Source: CAD feature listing. Evaluate the final solid. Frame: model axes, mm. A direction names the side the tool comes from. Round coordinates to 2 decimals unless told otherwise and drop trailing zeros. Order: outer loops, then holes, each group sorted by start corner. A loop starts at its lowest first (then second) coordinate and runs counter-clockwise, first axis right, second up. Notation, with made-up numbers: (10, -33.5) -> (58, -33.5) arc R17 ccw to (58, -4.5) -> close; hole circle Ø5 at (37.5, 16). An arc over 180 degrees is marked (long way). Write item = value, one per line. Start each with the question number.
(1) Cut plane B-B on y = 6. Return the cut outline in (x, z), then the cut area to 3 significant figures.
(2) Reachability of faces 4 (the face through (-16.296, 1.164, 45.286)), 5 (the face through (-7.105, 0.76, 41.004)), 6 (the face through (-4, 14.353, 14)), 7 (the face through (-4, -26.247, 14)), 8 (the face through (-14.208, -6, 19)) from +Z, -Z, +X, -X, +Y, -Y: full face, straight path, thin tool, end or side. Return the list, or none.
(3) Cut plane A-A on x = 1.25. Return the cut outline in (y, z).
(4) Cut plane D-D on z = 29.5. Return the cut outline in (x, y), then the cut area to 3 significant figures.
(5) Ray query, line 1 (Z direction, x = 0.5, y = -9.5); line 2 (Y direction, x = -10, z = 4); line 3 (Z direction, x = -13, y = -16). Return the intervals inside material, ascending.
(6) Cut plane C-C on y = -28.5. Return the cut outline in (x, z).
(7) Draft query along Y for faces 1 (the face through (-2, -2, 44.3)), 2 (the face through (-4, 20.753, 29)), 3 (the face through (1.305, -32.344, 28.972)). Return one class per face: released by +Y, released by -Y, zero draft, split by the parting line, or undercut.
(8) Contact query for flat-ended pins moving along their axis: pin 1 Ø5 at (x, z) = (-7.5, 9.5) entering from -Y; pin 2 Ø6 at (x, y) = (-10.41, 18.25) entering from -Z; pin 3 Ø1.5 at (y, z) = (-14, 34) entering from +X; pin 4 Ø3.5 at (x, y) = (1.79, -30.15) entering from -Z. Output: stop coordinate, or through.
from build123d import *

# Parameters (mm, degrees)
F0_W      = 19.8
F0_H      = 40.6
F1_DEPTH  = 27
F2_W      = 19.8
F2_H      = 6.4
F2_R      = 2.25
F3_DEPTH  = 4
F1_FACE_W = 19.8
F1_FACE_H = 40.6
F4_DEPTH  = 10.8
F5_SIZE   = 1
F6_R      = 2.8
F7_DEPTH  = 6.5
F8_R      = 12
F8_R_2    = 2.8
F9_DEPTH  = 2


with BuildPart() as f1:
    # F0 (on Top) → F1 (new body)
    with BuildSketch(Plane.XY):
        with Locations((-4.307641, -5.947228)):
            Rectangle(F0_W, F0_H)
    extrude(amount=F1_DEPTH)

    # F2 (on face) → F3 (join)
    with BuildSketch(Plane.XY.offset(27)):
        with Locations((-4.307641, 17.552772)):
            Rectangle(F2_W, F2_H)
        with Locations((-10.407641, 18.252772)):
            Circle(F2_R, mode=Mode.SUBTRACT)
        with Locations((1.792359, 18.252772)):
            Circle(F2_R, mode=Mode.SUBTRACT)
        with Locations((-4.307641, -29.447228)):
            Rectangle(F2_W, F2_H)
        with Locations((-10.407641, -30.147228)):
            Circle(F2_R, mode=Mode.SUBTRACT)
        with Locations((1.792359, -30.147228)):
            Circle(F2_R, mode=Mode.SUBTRACT)
    extrude(amount=F3_DEPTH)

    # F1_face (on face) → F4 (join)
    with BuildSketch(Plane(origin=(-4.307641, -5.947228, 27), x_dir=(1, 0, 0), z_dir=(0, 0, 1))):
        Rectangle(F1_FACE_W, F1_FACE_H)
    extrude(amount=F4_DEPTH)

    # F5
    f5_edges = [f1.edges().sort_by_distance(p)[0] for p in [
        (-14.207641, -5.947228, 0),
        (-4.307641, 14.352772, 0),
        (5.592359, -5.947228, 0),
        (-4.307641, -26.247228, 0),
    ]]
    chamfer(f5_edges, length=F5_SIZE)

    # F6 (on face) → F7 (join)
    with BuildSketch(Plane.XY.offset(37.8)):
        with Locations((-4.307641, 0.636772)):
            Circle(F6_R)
    extrude(amount=F7_DEPTH)

    # F8 (on face) → F9 (join)
    with BuildSketch(Plane.XY.offset(44.3)):
        with Locations((-4.307641, 0.636772)):
            Circle(F8_R)
        with Locations((-4.307641, 0.636772)):
            Circle(F8_R_2, mode=Mode.SUBTRACT)
        with Locations((-4.307641, 0.636772)):
            Circle(F8_R_2)
    extrude(amount=F9_DEPTH)


solid = f1.part
Evaluation:
q1.outline = (-15.04, 44.3) -> (6.43, 44.3) -> (6.43, 46.3) -> (-15.04, 46.3) -> close; (-14.21, 1) -> (-13.21, 0) -> (4.59, 0) -> (5.59, 1) -> (5.59, 37.8) -> (-14.21, 37.8) -> close
q1.area = 790 mm^2
q2.face_4 = +Z
q2.face_5 = none
q2.face_6 = -Z, +X, -X, +Y
q2.face_7 = -Z, +X, -X, -Y
q2.face_8 = -Z, -X, +Y, -Y
q3.outline = (-32.65, 27) -> (-32.33, 27) -> (-32.33, 31) -> (-32.65, 31) -> close; (-27.96, 27) -> (-26.25, 27) -> (-26.25, 1) -> (-25.25, 0) -> (13.35, 0) -> (14.35, 1) -> (14.35, 27) -> (16.07, 27) -> (16.07, 31) -> (14.35, 31) -> (14.35, 37.8) -> (-26.25, 37.8) -> (-26.25, 31) -> (-27.96, 31) -> close; (-10, 44.3) -> (11.27, 44.3) -> (11.27, 46.3) -> (-10, 46.3) -> close; (20.44, 27) -> (20.75, 27) -> (20.75, 31) -> (20.44, 31) -> close
q4.outline = (-14.21, -32.65) -> (5.59, -32.65) -> (5.59, 20.75) -> (-14.21, 20.75) -> close; hole circle Ø4.5 at (-10.41, -30.15); hole circle Ø4.5 at (-10.41, 18.25); hole circle Ø4.5 at (1.79, -30.15); hole circle Ø4.5 at (1.79, 18.25)
q4.area = 994 mm^2
q5.line_1 = 0 to 37.8, 44.3 to 46.3
q5.line_2 = -26.25 to 14.35
q5.line_3 = 0 to 37.8
q6.outline = (-14.21, 27) -> (-11.94, 27) -> (-11.94, 31) -> (-14.21, 31) -> close; (-8.87, 27) -> (0.26, 27) -> (0.26, 31) -> (-8.87, 31) -> close; (3.33, 27) -> (5.59, 27) -> (5.59, 31) -> (3.33, 31) -> close
q7.face_1 = zero draft
q7.face_2 = released by +Y
q7.face_3 = undercut
q8.pin_1 = -26.25
q8.pin_2 = 27
q8.pin_3 = 5.59
q8.pin_4 = through
